For this review, use the dimensioned drawing (mm, ordinates from the lowest corner) and the shaded views. Round coordinates to 2 decimals unless told otherwise and drop trailing zeros. Loops run counter-clockwise (first coordinate to the right, second up) from the corner with the lowest first, then second, coordinate; pieces in that order, holes last. Notation, with made-up numbers: M -24.5,36.25 L 17.5,36.25 A21 ccw 17.5,58.25 Z; hole C 3.5,0.25 d7. An arc over 180 degrees is marked long. Write item = value, one per line. Start each with the question number.
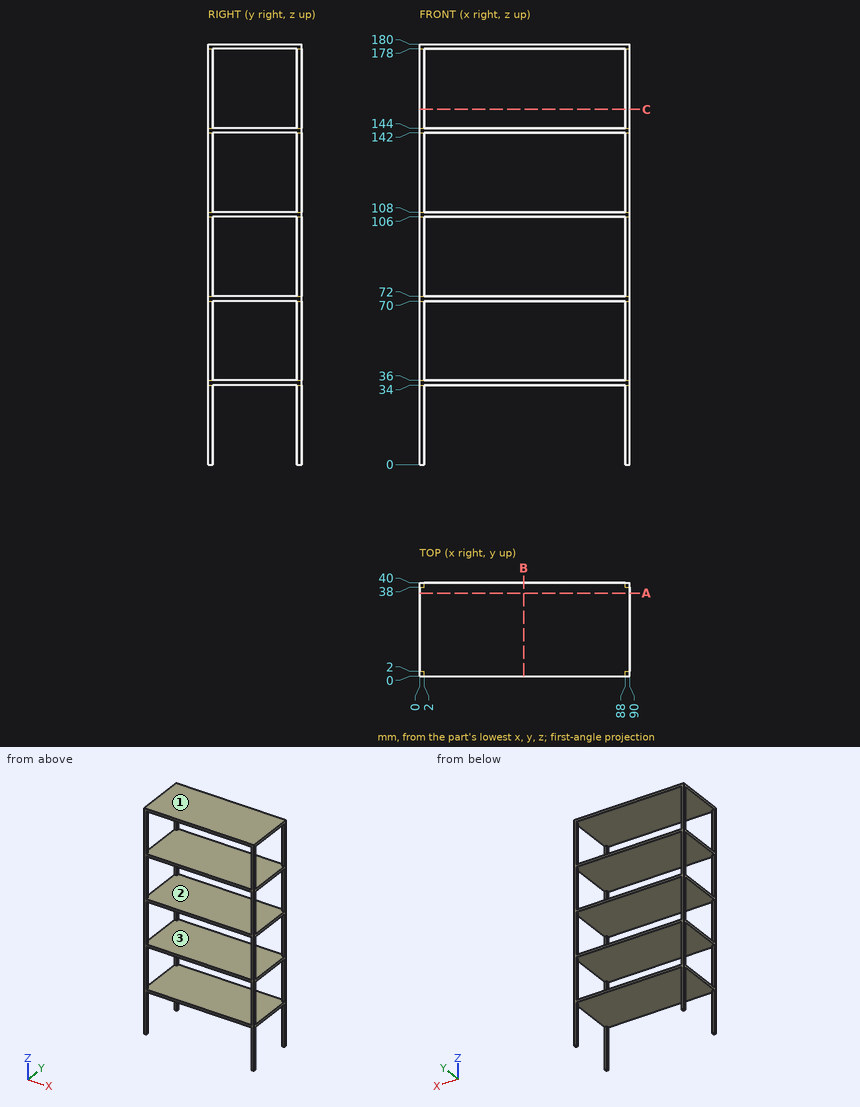
(1) Draft analysis for pull direction Z (two halves, no side actions). For the marked faces 1, 2 and 3, state which applies: +Z half, -Z half, draft (parallel to the pull), parting line (faces both ways), or undercut.
(2) Add section B-B on x = 44.5. Write out the cut boundary in (y, z), and give its area (3 significant figures).
(3) For pin 1 Ø12 at (x, y) = (34.5, 21.5) entering from -Z, flat-tipped, find the tip position at first contact; note if it passes through.
(4) Add section C-C on z = 152. Write out the cut boundary in (x, y), and give its area (3 significant figures).
(5) Wall thickness on L1, parallel to Z at x = 19.5, y = 8.5: over which ranges is the line inside the solid? List them lowest first.
(6) Add section A-A on y = 35.5. Write out the cut boundary in (x, z), and give its area (3 significant figures).
Answer sheet:
q1.face_1 = +Z half
q1.face_2 = undercut
q1.face_3 = undercut
q2.outline = M 0,34 L 40,34 L 40,36 L 0,36 Z; M 0,70 L 40,70 L 40,72 L 0,72 Z; M 0,106 L 40,106 L 40,108 L 0,108 Z; M 0,142 L 40,142 L 40,144 L 0,144 Z; M 0,178 L 40,178 L 40,180 L 0,180 Z
q2.area = 400 mm²
q3.pin_1 = 34
q4.outline = M 0,0 L 2,0 L 2,2 L 0,2 Z; M 0,38 L 2,38 L 2,40 L 0,40 Z; M 88,0 L 90,0 L 90,2 L 88,2 Z; M 88,38 L 90,38 L 90,40 L 88,40 Z
q4.area = 16.0 mm²
q5.L1 = 34 to 36, 70 to 72, 106 to 108, 142 to 144, 178 to 180
q6.outline = M 0,34 L 90,34 L 90,36 L 0,36 Z; M 0,70 L 90,70 L 90,72 L 0,72 Z; M 0,106 L 90,106 L 90,108 L 0,108 Z; M 0,142 L 90,142 L 90,144 L 0,144 Z; M 0,178 L 90,178 L 90,180 L 0,180 Z
q6.area = 900 mm²
